Geometry: final body of the model. Coordinates: model frame, mm. Face numbers are marked on the shaded views. A direction names the side the tool comes from. Coordinates: 2 decimals unless noted, no trailing zeros. Loops run counter-clockwise (first coordinate to the right, second up) from the corner with the lowest first, then second, coordinate; pieces in that order, holes last. Notation, with made-up numbers: (-3.75, 53) - (33.25, 53) arc R26 cw to (33.25, 71) - close; hole circle Ø11 at (49, 21.5). An arc over 180 degrees is marked (long way). Answer in a Markdown table with one row per item.
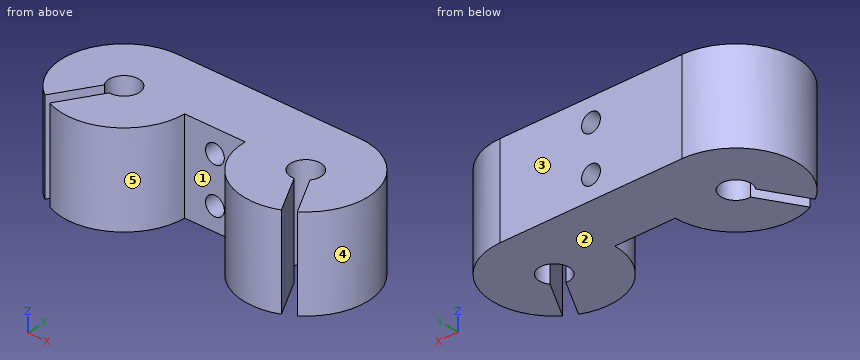
from build123d import *

# Parameters (mm, degrees)
BOSS_EXTRUDE1_DEPTH             = 15
SKETCH3_R                       = 2.45
CUT_EXTRUDE1_DEPTH              = 31.822070015
CUT_EXTRUDE2_DEPTH              = 31.822070015
F_3_0MM_CLEARANCE_DOWEL_HOLE1_D = 3.108


with BuildPart() as part:
    # Sketch2 → Boss-Extrude1 (new body)
    with BuildSketch(Plane.XY):
        with BuildLine():
            Line((-5, 10), (-15, 10))
            ThreePointArc((-15, 10), (-22.071067812, -7.071067812), (-5, 0))
            Line((-5, 0), (5, 0))
            ThreePointArc((5, 0), (22.071067812, -7.071067812), (15, 10))
            Line((15, 10), (5, 10))
            Line((5, 10), (-5, 10))
        make_face()
    extrude(amount=BOSS_EXTRUDE1_DEPTH)

    # Sketch3 → Cut-Extrude1 (cut, through all)
    with BuildSketch(Plane.XY.offset(15)):
        with Locations((-15, 0)):
            Circle(SKETCH3_R)
        with Locations((15, 0)):
            Circle(SKETCH3_R)
    extrude(amount=-CUT_EXTRUDE1_DEPTH, mode=Mode.SUBTRACT)

    # Sketch4 → Cut-Extrude2 (cut, through all)
    with BuildSketch(Plane.XY.offset(15)):
        Polygon((-14.133974596, -0.5), (-15.866025404, 0.5), (-20.866025404, -8.160254038), (-19.133974596, -9.160254038), align=None)
        Polygon((14.133974596, -0.5), (15.866025404, 0.5), (20.866025404, -8.160254038), (19.133974596, -9.160254038), align=None)
    extrude(amount=-CUT_EXTRUDE2_DEPTH, mode=Mode.SUBTRACT)

    # Ø3.0mm Clearance Dowel Hole1 (through all)
    with Locations(Plane(origin=(0, 0, 0), x_dir=(-1, 0, 0), z_dir=(0, -1, 0))):
        with Locations((0, -3.75), (0, -11.25)):
            Hole(F_3_0MM_CLEARANCE_DOWEL_HOLE1_D / 2)


solid = part.part
(1) Ray query, probe 1 along Z at (x, y) = (0, 5); probe 2 along Y at (x, z) = (-15, 10.75); probe 3 along X at (y, z) = (-1.5, 9). Return the intervals inside material, ascending.
Verdict:
| item | result |
|---|---|
| probe 1 | z = 0 to 2.2, 5.3 to 9.7, 12.8 to 15 |
| probe 2 | y = -10 to -2.45, 2.45 to 10 |
| probe 3 | x = -24.89 to -17.02, -13.06 to -5.11, 5.11 to 13.06, 17.02 to 24.89 |
(2) Cut plane A-A on x = 0. Output: boundary loops of the cut face in (y, z).
Verdict:
| item | result |
|---|---|
| outline | (0, 0) - (10, 0) - (10, 2.2) - (0, 2.2) - close; (0, 5.3) - (10, 5.3) - (10, 9.7) - (0, 9.7) - close; (0, 12.8) - (10, 12.8) - (10, 15) - (0, 15) - close |
(3) First-contact query: pin 1 Ø4 at (y, z) = (6, 7.5) entering from -X; pin 2 Ø3 at (x, z) = (-5.5, 7.5) entering from -Y; pin 3 Ø3 at (x, z) = (-0.5, 9) entering from -Y. Flat tips, straight axial feed; report the tip coordinate or a pass-through.
Verdict:
| item | result |
|---|---|
| pin 1 | stops at x = -24.17 |
| pin 2 | stops at y = -6 |
| pin 3 | stops at y = 0 |
(4) Cut plane B-B on z = 11.25. Output: boundary loops of the cut face in (x, y).
Verdict:
| item | result |
|---|---|
| outline | (-20.84, -8.12) - (-16.98, -1.44) arc R2.45 cw (long way) to (-15.25, -2.44) - (-19.11, -9.12) arc R10 ccw to (-5, 0) - (-1.55, 0) - (-1.55, 10) - (-15, 10) arc R10 ccw to start; (1.55, 0) - (5, 0) arc R10 ccw to (19.11, -9.12) - (15.25, -2.44) arc R2.45 cw (long way) to (16.98, -1.44) - (20.84, -8.12) arc R10 ccw to (15, 10) - (1.55, 10) - close |
(5) Cut plane C-C on y = -5.25. Output: boundary loops of the cut face in (x, z), then the cut area to 3 significant figures.
Verdict:
| item | result |
|---|---|
| outline | (-23.51, 0) - (-19.19, 0) - (-19.19, 15) - (-23.51, 15) - close; (-16.88, 0) - (-6.49, 0) - (-6.49, 15) - (-16.88, 15) - close; (6.49, 0) - (16.88, 0) - (16.88, 15) - (6.49, 15) - close; (19.19, 0) - (23.51, 0) - (23.51, 15) - (19.19, 15) - close |
| area | 441 mm² |
(6) Cut plane D-D on y = 1.75. Output: boundary loops of the cut face in (x, z).
Verdict:
| item | result |
|---|---|
| outline | (-24.85, 0) - (-16.71, 0) - (-16.71, 15) - (-24.85, 15) - close; (-13.29, 0) - (13.29, 0) - (13.29, 15) - (-13.29, 15) - close; (16.71, 0) - (24.85, 0) - (24.85, 15) - (16.71, 15) - close; hole circle Ø3.11 at (0, 3.75); hole circle Ø3.11 at (0, 11.25) |
(7) Access query for the marked faces 1 and 2. Directions: +Z, -Z, +X, -X, +Y, -Y. A direction counts if a zero-diameter tool reaches every point of the face in a straight line with its end or side. Return the directions, or none.
Verdict:
| item | result |
|---|---|
| face 1 | +Z, -Z, -Y |
| face 2 | -Z, +X, -X, +Y, -Y |
(8) Pull-direction query (X, two-part tool) for the marked faces 3, 4 and 5; classes: pulls with the +X half, pulls with the -X half, needs draft (parallel to the pull), parting line crosses it, or undercut.
Verdict:
| item | result |
|---|---|
| face 3 | needs draft |
| face 4 | pulls with the +X half |
| face 5 | undercut |
